Autodesk Fusion 360 part; units mm, degrees
sketch "Sketch1" plane through (0, 0, 7) normal (0, 0, 1) x (-1, 0, 0)
sketch "Sketch2" plane through (0, 0, 0) normal (0, 0, 1) x (1, 0, 0) in component "Bearing Bracket"
  point P0 (0, 65)
  dimension "d2" = 65
sketch "Sketch3" plane through (0, 0, 7) normal (0, 0, 1) x (-1, 0, 0) in component "Bearing Bracket"
  circle A0 centre (-17, -32.5) radius 4
  circle A1 centre (-64.9939, -32.5034) radius 11
  circle A2 centre (-117, -32.5) radius 4
  arc A3 (-134, -57) -> (-126, -65) centre (-126, -57) ccw
  line L0 (-126, -65) -> (-8, -65)
  arc A4 (-8, -65) -> (0, -57) centre (-8, -57) ccw
  line L1 (0, -57) -> (0, 0)
  line L2 (0, 0) -> (-134, 0)
  line L3 (-134, 0) -> (-134, -57)
  circle A5 centre (-64.9939, -32.5034) radius 10.5
  dimension "d3" = -0.5
extrude "Extrude1" add sketch "Sketch3" against normal blind 7 contours A3 L0 A4 L1 L2 L3
chamfer "Chamfer1" distance 0.2 angle 45 3 edges at (120.7293, 31.0535, 7) (75.2495, 28.5256, 7) (20.7293, 31.0535, 7)
chamfer "Chamfer2" distance 0.2 angle 45 1 edges at (20.7293, 33.9465, 0)
chamfer "Chamfer3" distance 0.2 angle 45 1 edges at (120.7293, 33.9465, 0)
chamfer "Chamfer4" distance 0.5 angle 45 6 edges at (134, 28.5, 0) (0, 28.5, 0) (2.3431, 62.6569, 0) (67, 65, 0) (131.6569, 62.6569, 0) (67, 0, 0)
chamfer "Chamfer5" distance 0.5 angle 45 6 edges at (0, 28.5, 7) (134, 28.5, 7) (131.6569, 62.6569, 7) (67, 65, 7) (2.3431, 62.6569, 7) (67, 0, 7)
sketch "Sketch2 (2)" plane through (0, 0, 7) normal (0, 0, 1) x (-1, 0, 0)
  circle A0 centre (-17, -32.5) radius 4.2
  circle A1 centre (-117, -32.5) radius 4.2
  circle A2 centre (-64.9939, -32.5034) radius 11.2
  line L0 (-133.5, -0.5) -> (-133.5, -57)
  arc A3 (-133.5, -57) -> (-126, -64.5) centre (-126, -57) ccw
  line L1 (-126, -64.5) -> (-8, -64.5)
  arc A4 (-8, -64.5) -> (-0.5, -57) centre (-8, -57) ccw
  line L2 (-0.5, -57) -> (-0.5, -0.5)
  line L3 (-0.5, -0.5) -> (-133.5, -0.5)
  circle A5 centre (-17, -32.5) radius 8
  circle A6 centre (-117, -32.5) radius 8
  line L4 (-117, -32.5) -> (-117, -44.5)
  line L5 (-117, -32.5) -> (-117, -20.5)
  line L6 (-117, -32.5) -> (-105, -32.5)
  line L7 (-117, -32.5) -> (-129, -32.5)
  circle A7 centre (-117, -44.5) radius 2
  circle A8 centre (-129, -32.5) radius 2
  circle A9 centre (-117, -20.5) radius 2
  circle A10 centre (-105, -32.5) radius 2
  line L8 (-17, -32.5) -> (-17, -44.5)
  line L9 (-17, -32.5) -> (-17, -20.5)
  line L10 (-17, -32.5) -> (-29, -32.5)
  line L11 (-17, -32.5) -> (-5, -32.5)
  circle A11 centre (-17, -44.5) radius 2
  circle A12 centre (-17, -20.5) radius 2
  circle A13 centre (-29, -32.5) radius 2
  circle A14 centre (-5, -32.5) radius 2
  dimension "d11" = 16
  dimension "d12" = 16
  dimension "d13" = 12
  dimension "d14" = 12
  dimension "d15" = 12
  dimension "d16" = 12
  dimension "d17" = 4
  dimension "d18" = 4
  dimension "d19" = 4
  dimension "d20" = 4
  dimension "d21" = 12
  dimension "d22" = 12
  dimension "d23" = 12
  dimension "d24" = 12
  dimension "d25" = 4
  dimension "d26" = 4
  dimension "d27" = 4
  dimension "d28" = 4
extrude "Extrude2" cut sketch "Sketch2 (2)" against normal blind 25 contours A0 L9 L11 | A0 A5 L8 L11 | A0 L8 L11 | A0 A5 L9 L11 | A0 L9 L10 | A0 A5 L9 L10 | A0 A5 L8 L10 | A0 L8 L10 | A11 | A13 | A12 | A14 | A1 L5 L6 | A1 A6 L4 L6 | A1 L4 L6 | A1 A6 L5 L6 | A1 L5 L7 | A1 A6 L5 L7 | A1 A6 L4 L7 | A1 L4 L7 | A7 | A8 | A9 | A10
chamfer "Chamfer6" distance 0.3 angle 45 1 edges at (124.4586, 29.6071, 7)
chamfer "Chamfer7" distance 0.2 angle 45 1 edges at (118.8647, 43.7768, 7)
chamfer "Chamfer8" distance 0.2 angle 45 1 edges at (124.7383, 35.5014, 7)
chamfer "Chamfer9" distance 0.2 angle 45 1 edges at (130.8647, 31.7768, 7)
chamfer "Chamfer10" distance 0.2 angle 45 1 edges at (118.8647, 19.7768, 7)
chamfer "Chamfer11" distance 0.2 angle 45 1 edges at (106.8647, 31.7768, 7)
chamfer "Chamfer12" distance 0.2 angle 45 5 edges at (24.4586, 29.6071, 7) (30.8647, 31.7768, 7) (18.8647, 43.7768, 7) (6.8647, 31.7768, 7) (18.8647, 19.7768, 7)
chamfer "Chamfer13" distance 0.2 angle 45 10 edges at (24.4586, 35.3929, 0) (6.8647, 33.2232, 0) (18.8647, 45.2232, 0) (30.8647, 33.2232, 0) (18.8647, 21.2232, 0) (118.8647, 21.2232, 0) (124.4586, 35.3929, 0) (106.8647, 33.2232, 0) (118.8647, 45.2232, 0) (130.8647, 33.2232, 0)
component "Bearing Bracket" placed x (1, 0, 0) y (0, 1, 0) z (0, 0, 1) at (0, 0, 0)
Model file for the job. Use its own axes, mm. Coordinates: 2 decimals unless noted, no trailing zeros. Write each loop counter-clockwise with the first axis right and the second up, starting at its lowest first coordinate (ties: lowest second). Pieces come first, ordered by that corner, then holes. Notation, with made-up numbers: (37.5, 85) - (61.5, 85) arc R19 ccw to (61.5, 94) - close; hole circle Ø7 at (62.25, 37). An arc over 180 degrees is marked (long way). One line per question, with ' | ' between items. Start each with the question number.
Q1. Cut at B-B, the plane x = 29. List the corners of the cut face in (y, z).
Q2. Drill centre lines: line 1 (Y direction, x = 117, z = 5); line 2 (X direction, y = 44.5, z = 2); line 3 (X direction, y = 29, z = 2.5). Where is each one in solid material? Low to high. Write a range as [from, to].
Q3. Pull direction X, two halves, no side cores. Call faces 1 (the face through (68, 65, 4)), 2 (the face through (5.434, 34.452, 3.546)), 3 (the face through (2.66, 62.46, 0.14)): pulls with the +X half, pulls with the -X half, needs draft (parallel to the pull), parting line crosses it, or undercut.
Q4. Cut at A-A, the plane x = 117. Give the number of separate pieces and of enclosed holes in the cut face, then the cut area to 3 significant figures.
Answer below:
1) outline: (0, 0.5) - (0.5, 0) - (30.3, 0) - (30.5, 0.2) - (30.5, 6.8) - (30.3, 7) - (0.5, 7) - (0, 6.5) - close; (34.5, 0.2) - (34.7, 0) - (64.5, 0) - (65, 0.5) - (65, 6.5) - (64.5, 7) - (34.7, 7) - (34.5, 6.8) - close
2) line 1: [0, 18.5], [22.5, 24.5], [40.5, 42.5], [46.5, 65] | line 2: [0, 15], [19, 115], [119, 134] | line 3: [0, 9.81], [24.19, 54.57], [75.42, 109.81], [124.19, 134]
3) face 1: needs draft | face 2: undercut | face 3: pulls with the -X half
4) separate pieces: 4 | enclosed holes: 0 | area: 286 mm^2
